Part model, mm, in its own coordinate system. A direction names the side the tool comes from. Round coordinates to 2 decimals unless told otherwise and drop trailing zeros. Loops run counter-clockwise (first coordinate to the right, second up) from the corner with the lowest first, then second, coordinate; pieces in that order, holes last. Notation, with made-up numbers: (29, -33) - (53, -33) arc R29 cw to (53, -10) - close; hole circle Ø2 at (87, 31). An arc over 180 degrees is marked (long way). Put each result on its own line as item: value.
from build123d import *

# Parameters (mm, degrees)
BOSS_EXTRUDE2_DEPTH = 25
BOSS_EXTRUDE3_DEPTH = 45
SKETCH3_W           = 15
SKETCH3_H           = 25
BOSS_EXTRUDE4_DEPTH = 25
SKETCH4_W           = 40
SKETCH4_H           = 30
CUT_EXTRUDE1_DEPTH  = 15
SKETCH5_R           = 11
CUT_EXTRUDE2_DEPTH  = 128.224012634


with BuildPart() as part:
    # Sketch1 → Boss-Extrude2 (new body)
    with BuildSketch(Plane.XY):
        Polygon((29.110234951, -15.315580854), (39.110234951, -15.315580854), (39.110234951, -2.038537921), (39.110234951, 14.698902507), (-50.889765049, 14.698902507), (-50.889765049, -2.301097493), (-15.889765049, -2.301097493), (-15.889765049, -7.315580854), (29.110234951, -7.315580854), align=None)
        with BuildLine():
            Line((-65.889765049, 12.698902507), (-65.889765049, 44.698902507))
            Line((-65.889765049, 44.698902507), (-50.889765049, 44.698902507))
            Line((-50.889765049, 44.698902507), (-50.889765049, 14.698902507))
            Line((-50.889765049, 14.698902507), (-50.889765049, -2.301097493))
            ThreePointArc((-50.889765049, -2.301097493), (-61.496366767, 2.092300789), (-65.889765049, 12.698902507))
        make_face()
    extrude(amount=-BOSS_EXTRUDE2_DEPTH)

    # Sketch2 → Boss-Extrude3 (add)
    with BuildSketch(Plane(origin=(0, 0, -25), x_dir=(-1, 0, 0), z_dir=(0, 0, -1))):
        Polygon((-39.110234951, -15.315580854), (-39.110234951, 14.698902507), (15.889765049, 14.698902507), (15.889765049, -2.301097493), (15.889765049, -7.315580854), (-29.110234951, -7.315580854), (-29.110234951, -15.315580854), align=None)
    extrude(amount=BOSS_EXTRUDE3_DEPTH)

    # Sketch3 → Boss-Extrude4 (add)
    with BuildSketch(Plane(origin=(0, 44.698902507, 0), x_dir=(1, 0, 0), z_dir=(0, 1, 0))):
        Polygon((-50.889765049, 25), (-50.889765049, 35.5), (-90.889765049, 35.5), (-90.889765049, -10.5), (-50.889765049, -10.5), (-50.889765049, 0), (-65.889765049, 0), (-65.889765049, 25), align=None)
        with Locations((-58.389765049, 12.5)):
            Rectangle(SKETCH3_W, SKETCH3_H)
    extrude(amount=BOSS_EXTRUDE4_DEPTH)

    # Sketch4 → Cut-Extrude1 (cut)
    with BuildSketch(Plane(origin=(0, 69.698902507, 0), x_dir=(1, 0, 0), z_dir=(0, 1, 0))):
        with Locations((-70.889765049, 12.5)):
            Rectangle(SKETCH4_W, SKETCH4_H)
    extrude(amount=-CUT_EXTRUDE1_DEPTH, mode=Mode.SUBTRACT)

    # Sketch5 → Cut-Extrude2 (cut, through all)
    with BuildSketch(Plane(origin=(0, 14.698902507, 0), x_dir=(1, 0, 0), z_dir=(0, 1, 0))):
        with Locations(Location((9.110234951, 18, 0), (0, 0, 180))):
            Circle(SKETCH5_R)
        with Locations(Location((9.110234951, 52, 0), (0, 0, 180))):
            Circle(SKETCH5_R)
    extrude(amount=-CUT_EXTRUDE2_DEPTH, mode=Mode.SUBTRACT)


solid = part.part
1. Tool access for faces 1 (the flat face through (6, -7.316, -35)), 2 (the flat face through (5, 14.699, -35)), 3 (the flat face through (-71, 54.699, -13)): list every direction of +Z, -Z, +X, -X, +Y, -Y with a clear straight run to the whole face (end or side of a thin tool).
A:
face 1: +Z, -Z, -X, -Y
face 2: +Z, -Z, +X, +Y
face 3: +X, -X, +Y
2. Band-saw the part on D-D (z = -18). List the corners of the cut face in (x, y).
A:
outline: (-90.89, 44.7) - (-65.89, 44.7) - (-65.89, 12.7) arc R15 ccw to (-50.89, -2.3) - (-15.89, -2.3) - (-15.89, -7.32) - (-1.89, -7.32) - (-1.89, 14.7) - (-50.89, 14.7) - (-50.89, 54.7) - (-90.89, 54.7) - close; (20.11, -7.32) - (29.11, -7.32) - (29.11, -15.32) - (39.11, -15.32) - (39.11, 14.7) - (20.11, 14.7) - close
3. Band-saw the part on A-A (z = -52). List the corners of the cut face in (x, y), plus the area to 3 significant figures.
A:
outline: (-15.89, -7.32) - (-1.89, -7.32) - (-1.89, 14.7) - (-15.89, 14.7) - close; (20.11, -7.32) - (29.11, -7.32) - (29.11, -15.32) - (39.11, -15.32) - (39.11, 14.7) - (20.11, 14.7) - close
area: 806 mm²
4. Band-saw the part on B-B (y = 7.5). List the corners of the cut face in (x, z), plus the area to 3 significant figures.
A:
outline: (-64.96, -25) - (-15.89, -25) - (-15.89, -70) - (39.11, -70) - (39.11, 0) - (-64.96, 0) - close; hole circle Ø22 at (9.11, -52); hole circle Ø22 at (9.11, -18)
area: 4,320 mm²
5. Band-saw the part on C-C (z = -1.5). List the corners of the cut face in (x, y), plus the area to 3 significant figures.
A:
outline: (-90.89, 44.7) - (-65.89, 44.7) - (-65.89, 12.7) arc R15 ccw to (-50.89, -2.3) - (-15.89, -2.3) - (-15.89, -7.32) - (29.11, -7.32) - (29.11, -15.32) - (39.11, -15.32) - (39.11, 14.7) - (-50.89, 14.7) - (-50.89, 54.7) - (-90.89, 54.7) - close
area: 2,940 mm²
6. Probe line 1 along Z through (x, y) = (6, 4); line 2 along Y through (x, z) = (-12.5, -50); line 3 along Z through (x, y) = (-59, 33). List the from-to ranges inside material, lowest first. Write a range as [from, to].
A:
line 1: z = [-70, -62.55], [-41.45, -28.55], [-7.45, 0]
line 2: y = [-7.32, 14.7]
line 3: z = [-25, 0]
7. Two-plate mould, pull along Z, no slides. Class faces 4 (the flat face through (-15.89, 4, -42)), 5 (the cylindrical face through (10.542, 3.846, -41.094)), 6 (the flat face through (-18, 10, 0)): pulls with the +Z half, pulls with the -Z half, needs draft (parallel to the pull), parting line crosses it, or undercut.
A:
face 4: needs draft
face 5: undercut
face 6: pulls with the +Z half
8. Pin check, flat tips, straight feed: P1, Ø14, axis at y = 42, z = -21.5, coming from the +X side; P2, Ø2, axis at x = -12.5, z = -56.5, coming from the +Y side; P3, Ø16.5, axis at x = -66, y = 62.5, coming from the -Z side. Stop position of each tip, or through.
A:
P1: stops at x = -50.89
P2: stops at y = 14.7
P3: stops at z = -35.5
